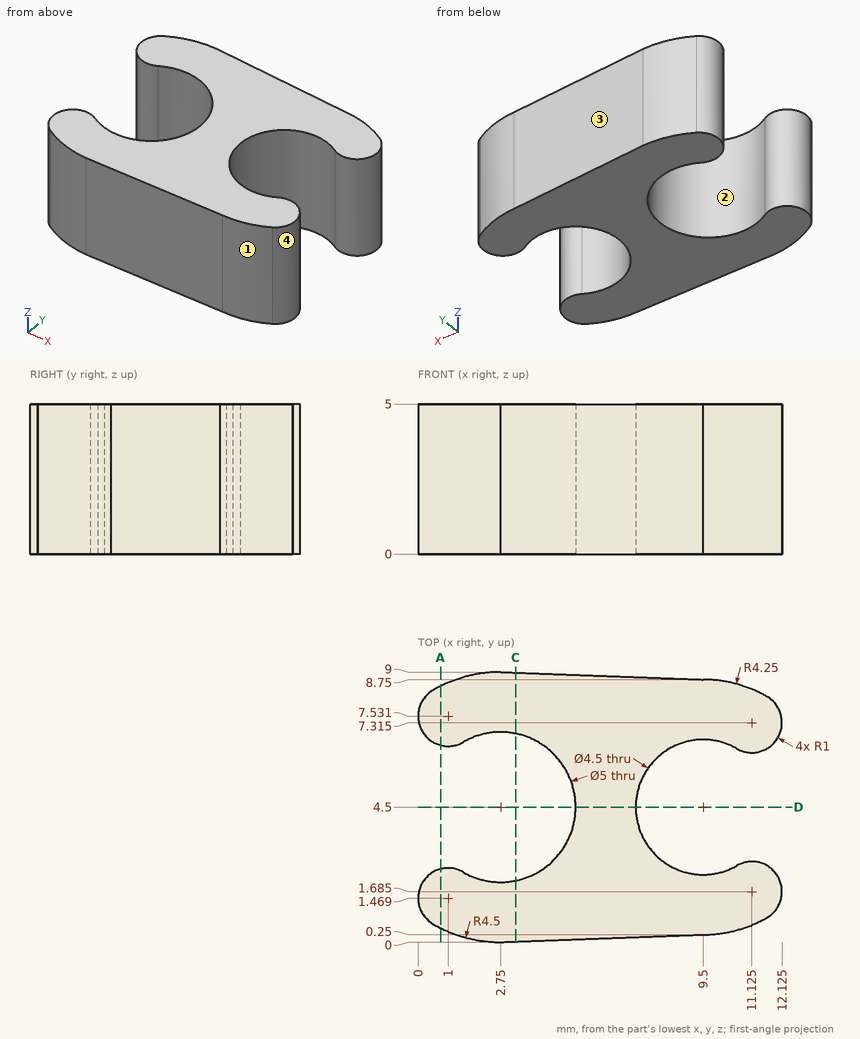
Design review of the part shown in the three views and the two pictorial views. Dimensions are in mm from the part's minimum x, y and z. Round coordinates to 2 decimals unless told otherwise and drop trailing zeros. Write each loop counter-clockwise with the first axis right and the second up, starting at its lowest first coordinate (ties: lowest second). Pieces come first, ordered by that corner, then holes. Notation, with made-up numbers: (75, 83) - (113, 83) arc R17 ccw to (113, 89) - close; hole circle Ø5 at (42.25, -36). An arc over 180 degrees is marked (long way). Return JSON: item names as keys, results as strings. Group by question number.
Item 1: We need section A-A on x = 0.75. Write out the cut boundary in (y, z).
Item 2: The part is to be moulded in two halves that separate along Y. For the marked faces 1, 2, 3 and 4, say which applies: pulls with the +Y half, pulls with the -Y half, needs draft (parallel to the pull), parting line crosses it, or undercut.
Item 3: We need section C-C on x = 3.25. Write out the cut boundary in (y, z), and give its area (3 significant figures).
Item 4: For probe 1 along Y at (x, z) = (2.75, 2.2); probe 2 along Y at (x, z) = (9.5, 2.3); probe 3 along Y at (x, z) = (5.5, 3.55), list the stretches that pass through material, from the lowest coordinate up. Write a range as [from, to].
Item 5: Insertion check: P1, Ø1, axis at x = 10.5, z = 2.5, coming from the -Y side. The pin has a flat end and moves straight along its axis. Give the tip position at first contact, or say it passes through.
Item 6: We need section D-D on y = 4.5. Write out the cut boundary in (x, z).
Model answer:
{
 "1": {"outline": "(0.47, 0) - (2.44, 0) - (2.44, 5) - (0.47, 5) - close; (6.56, 0) - (8.53, 0) - (8.53, 5) - (6.56, 5) - close"},
 "2": {"face 1": "pulls with the -Y half", "face 2": "undercut", "face 3": "pulls with the +Y half", "face 4": "undercut"},
 "3": {"outline": "(0.02, 0) - (2.05, 0) - (2.05, 5) - (0.02, 5) - close; (6.95, 0) - (8.98, 0) - (8.98, 5) - (6.95, 5) - close", "area": "20.3 mm²"},
 "4": {"probe 1": "y = [0, 2], [7, 9]", "probe 2": "y = [0.25, 2.25], [6.75, 8.75]", "probe 3": "y = [0.1, 8.9]"},
 "5": {"P1": "stops at y = 0.28"},
 "6": {"outline": "(5.25, 0) - (7.25, 0) - (7.25, 5) - (5.25, 5) - close"}
}
